```python
from build123d import *

# Parameters (mm, degrees)
CHAMFER1_SIZE  = 0.50801365
EXTRUDE1_REACH = 60.674
CHAMFER2_SIZE  = 1.524


with BuildPart() as part:
    # Sketch1 → Revolve1 (revolve)
    with BuildSketch(Plane(origin=(0, 0, 0), x_dir=(1, 0, 0), z_dir=(0, 1, 0)), mode=Mode.PRIVATE) as revolve1_sk:
        Polygon((7.366, -29.337), (7.366, 29.337), (3.1623, 29.337), (3.1623, 36.068), (0, 36.068), (0, -29.337), align=None)
    revolve(revolve1_sk.sketch.rotate(Axis((0, 0, -36.068), (0, 0, 1)), 180), axis=Axis((0, 0, -36.068), (0, 0, 1)))  # turned: the seam where the file's is

    # Chamfer1
    chamfer1_edges = [part.edges().sort_by_distance(p)[0] for p in [
        (3.1623, 0, -36.068),
    ]]
    chamfer(chamfer1_edges, length=CHAMFER1_SIZE)

    # Sketch2 → Extrude1 (cut, up to next)
    with BuildSketch(Plane(origin=(0, 0, -29.337), x_dir=(-1, 0, 0), z_dir=(0, 0, -1)), mode=Mode.PRIVATE) as extrude1_sk1:
        with BuildLine():
            ThreePointArc((3.683, 6.379143124), (0, 7.366), (-3.683, 6.379143124))
            Line((-3.683, 6.379143124), (3.683, 6.379143124))
        make_face()
    extrude1_tool1 = extrude(extrude1_sk1.sketch, amount=-EXTRUDE1_REACH, mode=Mode.PRIVATE) & part.part
    add(extrude1_tool1.solids().sort_by_distance((0, 6.776244, -29.337))[0], mode=Mode.SUBTRACT)
    # Sketch2 → Extrude1 (cut, up to next)
    with BuildSketch(Plane(origin=(0, 0, -29.337), x_dir=(-1, 0, 0), z_dir=(0, 0, -1)), mode=Mode.PRIVATE) as extrude1_sk2:
        with BuildLine():
            ThreePointArc((7.366, 0), (6.379143124, 3.683), (3.683, 6.379143124))
            Line((3.683, 6.379143124), (7.366, 0))
        make_face()
    extrude1_tool2 = extrude(extrude1_sk2.sketch, amount=-EXTRUDE1_REACH, mode=Mode.PRIVATE) & part.part
    add(extrude1_tool2.solids().sort_by_distance((-5.868399, 3.388122, -29.337))[0], mode=Mode.SUBTRACT)
    # Sketch2 → Extrude1 (cut, up to next)
    with BuildSketch(Plane(origin=(0, 0, -29.337), x_dir=(-1, 0, 0), z_dir=(0, 0, -1)), mode=Mode.PRIVATE) as extrude1_sk3:
        with BuildLine():
            Line((7.366, 0), (3.683, -6.379143124))
            ThreePointArc((3.683, -6.379143124), (6.379143124, -3.683), (7.366, 0))
        make_face()
    extrude1_tool3 = extrude(extrude1_sk3.sketch, amount=-EXTRUDE1_REACH, mode=Mode.PRIVATE) & part.part
    add(extrude1_tool3.solids().sort_by_distance((-5.868399, -3.388122, -29.337))[0], mode=Mode.SUBTRACT)
    # Sketch2 → Extrude1 (cut, up to next)
    with BuildSketch(Plane(origin=(0, 0, -29.337), x_dir=(-1, 0, 0), z_dir=(0, 0, -1)), mode=Mode.PRIVATE) as extrude1_sk4:
        with BuildLine():
            Line((3.683, -6.379143124), (-3.683, -6.379143124))
            ThreePointArc((-3.683, -6.379143124), (0, -7.366), (3.683, -6.379143124))
        make_face()
    extrude1_tool4 = extrude(extrude1_sk4.sketch, amount=-EXTRUDE1_REACH, mode=Mode.PRIVATE) & part.part
    add(extrude1_tool4.solids().sort_by_distance((0, -6.776244, -29.337))[0], mode=Mode.SUBTRACT)
    # Sketch2 → Extrude1 (cut, up to next)
    with BuildSketch(Plane(origin=(0, 0, -29.337), x_dir=(-1, 0, 0), z_dir=(0, 0, -1)), mode=Mode.PRIVATE) as extrude1_sk5:
        with BuildLine():
            Line((-3.683, -6.379143124), (-7.366, 0))
            ThreePointArc((-7.366, 0), (-6.379143124, -3.683), (-3.683, -6.379143124))
        make_face()
    extrude1_tool5 = extrude(extrude1_sk5.sketch, amount=-EXTRUDE1_REACH, mode=Mode.PRIVATE) & part.part
    add(extrude1_tool5.solids().sort_by_distance((5.868399, -3.388122, -29.337))[0], mode=Mode.SUBTRACT)
    # Sketch2 → Extrude1 (cut, up to next)
    with BuildSketch(Plane(origin=(0, 0, -29.337), x_dir=(-1, 0, 0), z_dir=(0, 0, -1)), mode=Mode.PRIVATE) as extrude1_sk6:
        with BuildLine():
            ThreePointArc((-3.683, 6.379143124), (-6.379143124, 3.683), (-7.366, 0))
            Line((-7.366, 0), (-3.683, 6.379143124))
        make_face()
    extrude1_tool6 = extrude(extrude1_sk6.sketch, amount=-EXTRUDE1_REACH, mode=Mode.PRIVATE) & part.part
    add(extrude1_tool6.solids().sort_by_distance((5.868399, 3.388122, -29.337))[0], mode=Mode.SUBTRACT)

    # Chamfer2
    chamfer2_edges = [part.edges().sort_by_distance(p)[0] for p in [
        (0, 6.379143124, -29.337),
        (-5.5245, 3.189571562, -29.337),
        (-5.5245, -3.189571562, -29.337),
        (0, -6.379143124, -29.337),
        (5.5245, -3.189571562, -29.337),
        (5.5245, 3.189571562, -29.337),
    ]]
    chamfer(chamfer2_edges, length=CHAMFER2_SIZE)


solid = part.part
```
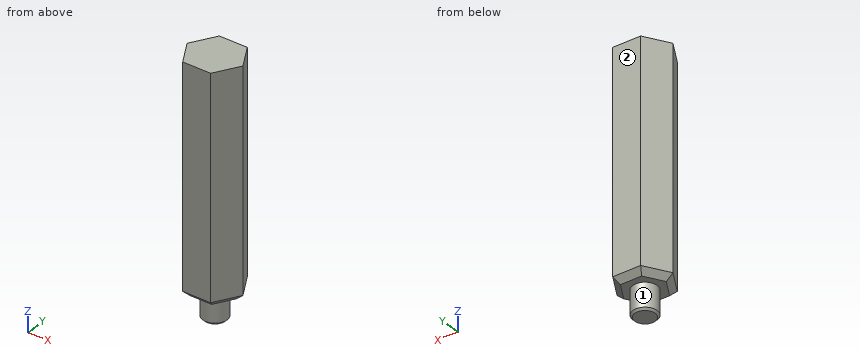
Geometry: final body of the model. Coordinates: model frame, mm. Face numbers are marked on the shaded views. A direction names the side the tool comes from. Round coordinates to 2 decimals unless told otherwise and drop trailing zeros. Loops run counter-clockwise (first coordinate to the right, second up) from the corner with the lowest first, then second, coordinate; pieces in that order, holes last. Notation, with made-up numbers: (64.25, 25.5) -> (106.25, 25.5) arc R18 ccw to (106.25, 39.5) -> close; hole circle Ø3 at (23, -7.5). An arc over 180 degrees is marked (long way). Use one line per item in the form item = value.
Item 1: Cut plane B-B on x = 0. Output: boundary loops of the cut face in (y, z).
Evaluation:
outline = (-6.38, -27.81) -> (-4.86, -29.34) -> (-3.16, -29.34) -> (-3.16, -35.56) -> (-2.65, -36.07) -> (2.65, -36.07) -> (3.16, -35.56) -> (3.16, -29.34) -> (4.86, -29.34) -> (6.38, -27.81) -> (6.38, 29.34) -> (-6.38, 29.34) -> close
Item 2: Cut plane C-C on y = 5.75. Output: boundary loops of the cut face in (x, z).
Evaluation:
outline = (-4.05, -27.81) -> (-3.32, -28.44) -> (3.32, -28.44) -> (4.05, -27.81) -> (4.05, 29.34) -> (-4.05, 29.34) -> close
Item 3: Material intervals for probe 1 along Z at (x, y) = (-1.5, 3); probe 2 along Z at (x, y) = (-1.5, -6); probe 3 along X at (y, z) = (-5.25, -19), sorted ascending.
Evaluation:
probe_1 = -29.34 to 29.34
probe_2 = -28.19 to 29.34
probe_3 = -4.33 to 4.33
Item 4: Cut plane A-A on z = -19.5. Output: boundary loops of the cut face in (x, y).
Evaluation:
outline = (-7.37, 0) -> (-3.68, -6.38) -> (3.68, -6.38) -> (7.37, 0) -> (3.68, 6.38) -> (-3.68, 6.38) -> close
Item 5: Contact query for a flat-ended pin moving along its axis: pin 1 Ø1 at (x, y) = (3, -4) entering from -Z. Output: stop coordinate, or through.
Evaluation:
pin_1 = -29.34
Item 6: Access query for the marked faces 1 and 2. Directions: +Z, -Z, +X, -X, +Y, -Y. A direction counts if a zero-diameter tool reaches every point of the face in a straight line with its end or side. Return the directions, or none.
Evaluation:
face_1 = -Z
face_2 = +Z, -Z, +X, -X, +Y
